Here's how the part is built. I have some questions about the finished solid (model axes, mm). Round coordinates to 2 decimals unless told otherwise and drop trailing zeros. Write each loop counter-clockwise with the first axis right and the second up, starting at its lowest first coordinate (ties: lowest second). Pieces come first, ordered by that corner, then holes. Notation, with made-up numbers: (-23.75, -28) - (-13.75, -28) arc R15 cw to (-13.75, -19) - close; hole circle Ø5 at (75, 19). An arc over 180 degrees is marked (long way). One line per item, written item: value. Start each with the question number.
Item 1: Imagine slicing it at C-C, the plane z = 22.5. Please give me the cut outline in (x, y), then the cut area to 3 significant figures.
Item 2: Imagine slicing it at B-B, the plane z = 126. Please give me the cut outline in (x, y), then the cut area to 3 significant figures.
Item 3: For P1, Ø6, axis at y = 12, z = 114, coming from the -X side; P2, Ø6, axis at y = 5.5, z = -110.5, coming from the +X side; P3, Ø10, axis at x = 142, y = 8, coming from the +Z side, each with a flat end and sliding along its axis, tell me the tip position at first contact or that it passes through.
Item 4: If I drill on line 1 (X direction, y = 3.5, z = -4); line 2 (X direction, y = 10.75, z = 54); line 3 (Z direction, x = 15, y = 16), over which ranges is the centre line in solid material (lowest first)?
Item 5: Imagine slicing it at A-A, the plane x = -24. Please give me the cut outline in (y, z), then the cut area to 3 significant figures.
Item 6: Imagine slicing it at D-D, the plane x = -113.5. Please give me the cut outline in (y, z), then the cut area to 3 significant figures.
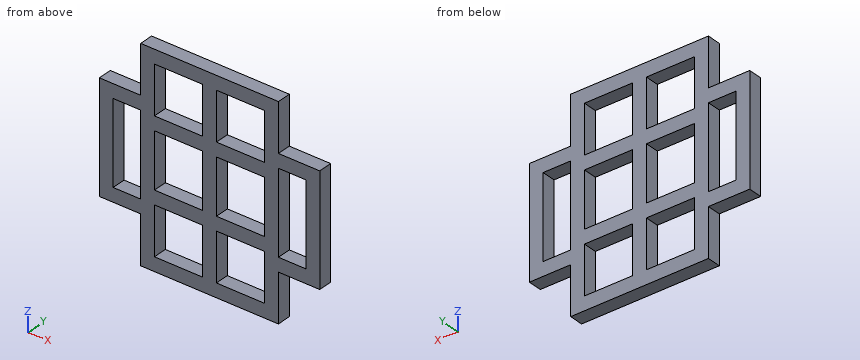
```python
from build123d import *

# Parameters (mm, degrees)
SKETCH4_W           = 70
SKETCH4_H           = 70
SKETCH4_H_2         = 80
SKETCH4_W_2         = 40
SKETCH4_H_3         = 120
BOSS_EXTRUDE2_DEPTH = 20


with BuildPart() as part:
    # Sketch4 → Boss-Extrude2 (new body)
    with BuildSketch(Plane(origin=(0, 0, 0), x_dir=(1, 0, 0), z_dir=(0, 1, 0))):
        Polygon((-100, 150), (100, 150), (100, 80), (160, 80), (160, -80), (100, -80), (100, -150), (-100, -150), (-100, -80), (-160, -80), (-160, 80), (-100, 80), align=None)
        with Locations((-45, 95)):
            Rectangle(SKETCH4_W, SKETCH4_H, mode=Mode.SUBTRACT)
        with Locations((45, 95)):
            Rectangle(SKETCH4_W, SKETCH4_H, mode=Mode.SUBTRACT)
        with Locations((-45, 0)):
            Rectangle(SKETCH4_W, SKETCH4_H_2, mode=Mode.SUBTRACT)
        with Locations((45, 0)):
            Rectangle(SKETCH4_W, SKETCH4_H_2, mode=Mode.SUBTRACT)
        with Locations((-45, -95)):
            Rectangle(SKETCH4_W, SKETCH4_H, mode=Mode.SUBTRACT)
        with Locations((45, -95)):
            Rectangle(SKETCH4_W, SKETCH4_H, mode=Mode.SUBTRACT)
        with Locations((120, 0)):
            Rectangle(SKETCH4_W_2, SKETCH4_H_3, mode=Mode.SUBTRACT)
        with Locations((-120, 0)):
            Rectangle(SKETCH4_W_2, SKETCH4_H_3, mode=Mode.SUBTRACT)
    extrude(amount=BOSS_EXTRUDE2_DEPTH)


solid = part.part
```
Values follow:
1. outline: (-160, 0) - (-140, 0) - (-140, 20) - (-160, 20) - close; (-100, 0) - (-80, 0) - (-80, 20) - (-100, 20) - close; (-10, 0) - (10, 0) - (10, 20) - (-10, 20) - close; (80, 0) - (100, 0) - (100, 20) - (80, 20) - close; (140, 0) - (160, 0) - (160, 20) - (140, 20) - close
1. area: 2,000 mm^2
2. outline: (-100, 0) - (-80, 0) - (-80, 20) - (-100, 20) - close; (-10, 0) - (10, 0) - (10, 20) - (-10, 20) - close; (80, 0) - (100, 0) - (100, 20) - (80, 20) - close
2. area: 1,200 mm^2
3. P1: stops at x = -100
3. P2: stops at x = 100
3. P3: stops at z = 80
4. line 1: x = -160 to -140, -100 to -80, -10 to 10, 80 to 100, 140 to 160
4. line 2: x = -160 to -140, -100 to 100, 140 to 160
4. line 3: z = -150 to -130, -60 to -40, 40 to 60, 130 to 150
5. outline: (0, -150) - (20, -150) - (20, -130) - (0, -130) - close; (0, -60) - (20, -60) - (20, -40) - (0, -40) - close; (0, 40) - (20, 40) - (20, 60) - (0, 60) - close; (0, 130) - (20, 130) - (20, 150) - (0, 150) - close
5. area: 1,600 mm^2
6. outline: (0, -80) - (20, -80) - (20, -60) - (0, -60) - close; (0, 60) - (20, 60) - (20, 80) - (0, 80) - close
6. area: 800 mm^2
